Input: part model. Units: mm. Frame: model coordinates. A direction names the side the tool comes from. Coordinates: 2 decimals unless noted, no trailing zeros. Write each loop counter-clockwise with the first axis right and the second up, starting at its lowest first coordinate (ties: lowest second). Pieces come first, ordered by that corner, then holes.
1) Section query B-B (y = -1). Output: boundary loops of the cut face in (x, z).
2) Pin query (flat end, axial travel): pin 1 Ø6.5 at (y, z) = (67.5, -52.5) entering from -X. Return the tip coordinate at first contact, or that it passes through.
3) Line query: L1, parallel to Z at x = 1.55, y = -185; L2, parallel to Z at x = -22, y = 141.5; L3, parallel to Y at x = -14.5, z = 13.5. Output: solid intervals per line, ascending.
4) Draft query along X for faces 4 (the flat face through (0.5, 185, -65)), 5 (the flat face through (-13, -3, -60)), 6 (the flat face through (0, -175, -54)), 7 (the flat face through (0.5, -185, -65)). Return one class per face: pulls with the +X half, pulls with the -X half, needs draft (parallel to the pull), parting line crosses it, or undercut.
5) Set-up query: faces 1 (the cylindrical face through (1.565, 188.075, 64.317)), 2 (the flat face through (-13, 190, -1)), 3 (the flat face through (0, -60, -54)). Return all of +Z, -Z, +X, -X, +Y, -Y with unobstructed straight access to the full face (end or side cutting, diameter ignored); none if empty.
6) Section query A-A (x = -18.5). Output: boundary loops of the cut face in (y, z).
7) Section query C-C (z = 17). Output: boundary loops of the cut face in (x, y), then the cut area to 3 significant figures.
from build123d import *

# Parameters (mm, degrees)
SKETCH1_W                        = 380
SKETCH1_H                        = 140
SKETCH1_W_2                      = 360
SKETCH1_H_2                      = 120
SKETCH1_R                        = 2
BOSS_EXTRUDE2_DEPTH              = 3
SKETCH1_6_W                      = 380
SKETCH1_6_H                      = 140
SKETCH1_6_W_2                    = 360
SKETCH1_6_H_2                    = 120
BOSS_EXTRUDE5_DEPTH              = 29
SKETCH14_W                       = 378
SKETCH14_H                       = 138
SKETCH14_W_2                     = 377.2
SKETCH14_H_2                     = 137.2
BOSS_EXTRUDE7_DEPTH              = 0.2
SKETCH14_4_R                     = 3.95
BOSS_EXTRUDE9_DEPTH              = 0.8
MOUNTING_MAGNET_HOLES_DEPTH      = 0.6
MOUNTING_MAGNET_HOLES_DEPTH_BACK = 1.5
SKETCH14_5_R                     = 3.15
SKETCH17_W                       = 378.4
SKETCH17_H                       = 138.4
SKETCH17_W_2                     = 377.2
SKETCH17_H_2                     = 137.2
BOSS_EXTRUDE10_DEPTH             = 0.4
CHAMFER1_SIZE                    = 0.4
CHAMFER1_SIZE_2                  = 0.230940108
COVER_START                      = -0.4
SKETCH18_R                       = 3.15
COVER_MAGNET_HOLES_DEPTH         = 2.1


with BuildPart() as part:
    # Sketch1 → Boss-Extrude2 (new body)
    # profile 1 of 13: a face of its own
    with BuildSketch(Plane.YZ):
        Rectangle(SKETCH1_W, SKETCH1_H)
        Rectangle(SKETCH1_W_2, SKETCH1_H_2, mode=Mode.SUBTRACT)
    # profile 2 of 13: a face of its own
    with BuildSketch(Plane.YZ):
        with BuildLine():
            Line((-180, 60), (-180, 48))
            Line((-180, 48), (-174, 48))
            ThreePointArc((-174, 48), (-169.757359313, 49.757359313), (-168, 54))
            Line((-168, 54), (-168, 60))
            Line((-168, 60), (-180, 60))
        make_face()
        with Locations(Location((-172.5, 52.5, 0), (0, 0, 270))):
            Circle(SKETCH1_R, mode=Mode.SUBTRACT)
    # profile 3 of 13: a face of its own
    with BuildSketch(Plane.YZ):
        with BuildLine():
            Line((-60, 60), (-72, 60))
            Line((-72, 60), (-72, 54))
            ThreePointArc((-72, 54), (-70.242640687, 49.757359313), (-66, 48))
            Line((-66, 48), (-60, 48))
            Line((-60, 48), (-60, 60))
        make_face()
        with Locations(Location((-67.5, 52.5, 0), (0, 0, 270))):
            Circle(SKETCH1_R, mode=Mode.SUBTRACT)
    # profile 4 of 13: a face of its own
    with BuildSketch(Plane.YZ):
        with BuildLine():
            Line((-48, 60), (-60, 60))
            Line((-60, 60), (-60, 48))
            Line((-60, 48), (-54, 48))
            ThreePointArc((-54, 48), (-49.757359313, 49.757359313), (-48, 54))
            Line((-48, 54), (-48, 60))
        make_face()
        with Locations(Location((-52.5, 52.5, 0), (0, 0, 270))):
            Circle(SKETCH1_R, mode=Mode.SUBTRACT)
    # profile 5 of 13: a face of its own
    with BuildSketch(Plane.YZ):
        with BuildLine():
            Line((-60, -48), (-60, -60))
            Line((-60, -60), (-48, -60))
            Line((-48, -60), (-48, -54))
            ThreePointArc((-48, -54), (-49.757359313, -49.757359313), (-54, -48))
            Line((-54, -48), (-60, -48))
        make_face()
        with Locations(Location((-52.5, -52.5, 0), (0, 0, 270))):
            Circle(SKETCH1_R, mode=Mode.SUBTRACT)
    # profile 6 of 13: a face of its own
    with BuildSketch(Plane.YZ):
        with BuildLine():
            Line((-72, -54), (-72, -60))
            Line((-72, -60), (-60, -60))
            Line((-60, -60), (-60, -48))
            Line((-60, -48), (-66, -48))
            ThreePointArc((-66, -48), (-70.242640687, -49.757359313), (-72, -54))
        make_face()
        with Locations(Location((-67.5, -52.5, 0), (0, 0, 270))):
            Circle(SKETCH1_R, mode=Mode.SUBTRACT)
    # profile 7 of 13: a face of its own
    with BuildSketch(Plane.YZ):
        with BuildLine():
            Line((-180, -48), (-180, -60))
            Line((-180, -60), (-168, -60))
            Line((-168, -60), (-168, -54))
            ThreePointArc((-168, -54), (-169.757359313, -49.757359313), (-174, -48))
            Line((-174, -48), (-180, -48))
        make_face()
        with Locations(Location((-172.5, -52.5, 0), (0, 0, 270))):
            Circle(SKETCH1_R, mode=Mode.SUBTRACT)
    # profile 8 of 13: a face of its own
    with BuildSketch(Plane.YZ):
        with BuildLine():
            Line((48, -54), (48, -60))
            Line((48, -60), (60, -60))
            Line((60, -60), (60, -48))
            Line((60, -48), (54, -48))
            ThreePointArc((54, -48), (49.757359313, -49.757359313), (48, -54))
        make_face()
        with Locations(Location((52.5, -52.5, 0), (0, 0, 270))):
            Circle(SKETCH1_R, mode=Mode.SUBTRACT)
    # profile 9 of 13: a face of its own
    with BuildSketch(Plane.YZ):
        with BuildLine():
            Line((60, -48), (60, -60))
            Line((60, -60), (72, -60))
            Line((72, -60), (72, -54))
            ThreePointArc((72, -54), (70.242640687, -49.757359313), (66, -48))
            Line((66, -48), (60, -48))
        make_face()
        with Locations(Location((67.5, -52.5, 0), (0, 0, 270))):
            Circle(SKETCH1_R, mode=Mode.SUBTRACT)
    # profile 10 of 13: a face of its own
    with BuildSketch(Plane.YZ):
        with BuildLine():
            Line((72, 60), (60, 60))
            Line((60, 60), (60, 48))
            Line((60, 48), (66, 48))
            ThreePointArc((66, 48), (70.242640687, 49.757359313), (72, 54))
            Line((72, 54), (72, 60))
        make_face()
        with Locations(Location((67.5, 52.5, 0), (0, 0, 270))):
            Circle(SKETCH1_R, mode=Mode.SUBTRACT)
    # profile 11 of 13: a face of its own
    with BuildSketch(Plane.YZ):
        with BuildLine():
            Line((60, 60), (48, 60))
            Line((48, 60), (48, 54))
            ThreePointArc((48, 54), (49.757359313, 49.757359313), (54, 48))
            Line((54, 48), (60, 48))
            Line((60, 48), (60, 60))
        make_face()
        with Locations(Location((52.5, 52.5, 0), (0, 0, 270))):
            Circle(SKETCH1_R, mode=Mode.SUBTRACT)
    # profile 12 of 13: a face of its own
    with BuildSketch(Plane.YZ):
        with BuildLine():
            Line((174, 48), (180, 48))
            Line((180, 48), (180, 60))
            Line((180, 60), (168, 60))
            Line((168, 60), (168, 54))
            ThreePointArc((168, 54), (169.757359313, 49.757359313), (174, 48))
        make_face()
        with Locations(Location((172.5, 52.5, 0), (0, 0, 270))):
            Circle(SKETCH1_R, mode=Mode.SUBTRACT)
    # profile 13 of 13: a face of its own
    with BuildSketch(Plane.YZ):
        with BuildLine():
            Line((168, -54), (168, -60))
            Line((168, -60), (180, -60))
            Line((180, -60), (180, -48))
            Line((180, -48), (174, -48))
            ThreePointArc((174, -48), (169.757359313, -49.757359313), (168, -54))
        make_face()
        with Locations(Location((172.5, -52.5, 0), (0, 0, 270))):
            Circle(SKETCH1_R, mode=Mode.SUBTRACT)
    extrude(amount=BOSS_EXTRUDE2_DEPTH)

    # Sketch1<6> → Boss-Extrude5 (add)
    with BuildSketch(Plane.YZ):
        Rectangle(SKETCH1_6_W, SKETCH1_6_H)
        Rectangle(SKETCH1_6_W_2, SKETCH1_6_H_2, mode=Mode.SUBTRACT)
    extrude(amount=-BOSS_EXTRUDE5_DEPTH)

    # Sketch14 → Boss-Extrude7 (add)
    with BuildSketch(Plane(origin=(-29, 0, 0), x_dir=(0, -1, 0), z_dir=(-1, 0, 0))):
        Rectangle(SKETCH14_W, SKETCH14_H)
        Rectangle(SKETCH14_W_2, SKETCH14_H_2, mode=Mode.SUBTRACT)
    extrude(amount=BOSS_EXTRUDE7_DEPTH)

    # Sketch14<4> → Boss-Extrude9 (add)
    with BuildSketch(Plane(origin=(-29, 0, 0), x_dir=(0, -1, 0), z_dir=(-1, 0, 0))):
        with Locations(Location((-182.928932188, 62.928932188, 0), (0, 0, 270))):
            Circle(SKETCH14_4_R)
        with Locations(Location((182.928932188, 62.928932188, 0), (0, 0, 270))):
            Circle(SKETCH14_4_R)
        with Locations(Location((182.928932188, -62.928932188, 0), (0, 0, 270))):
            Circle(SKETCH14_4_R)
        with Locations(Location((-182.928932188, -62.928932188, 0), (0, 0, 270))):
            Circle(SKETCH14_4_R)
    extrude(amount=BOSS_EXTRUDE9_DEPTH)

    # Sketch14<5> → Mounting magnet holes (cut, two sides: drawn at the far end of the back side and taken through both)
    with BuildSketch(Plane(origin=(-29, 0, 0), x_dir=(0, -1, 0), z_dir=(-1, 0, 0)).offset(-MOUNTING_MAGNET_HOLES_DEPTH_BACK)):
        with Locations(Location((-182.928932188, 62.928932188, 0), (0, 0, 90))):
            Circle(SKETCH14_5_R)
        with Locations(Location((182.928932188, 62.928932188, 0), (0, 0, 270))):
            Circle(SKETCH14_5_R)
        with Locations(Location((182.928932188, -62.928932188, 0), (0, 0, 90))):
            Circle(SKETCH14_5_R)
        with Locations(Location((-182.928932188, -62.928932188, 0), (0, 0, 270))):
            Circle(SKETCH14_5_R)
    extrude(amount=MOUNTING_MAGNET_HOLES_DEPTH + MOUNTING_MAGNET_HOLES_DEPTH_BACK, mode=Mode.SUBTRACT)

    # Sketch17 → Boss-Extrude10 (add)
    with BuildSketch(Plane(origin=(-29.2, 0, 0), x_dir=(0, -1, 0), z_dir=(-1, 0, 0))):
        Rectangle(SKETCH17_W, SKETCH17_H)
        Rectangle(SKETCH17_W_2, SKETCH17_H_2, mode=Mode.SUBTRACT)
    extrude(amount=BOSS_EXTRUDE10_DEPTH)

    # Chamfer1
    # the kernel refuses this chamfer: 0.4, 0.230940108 mm, written as the material it takes off along each edge
    with BuildSketch(Plane(origin=(-29.6, 190.234834302, -69.2), x_dir=(0.9998132206222082, 0, -0.01932676561269006), z_dir=(0, -1, 0))) as chamfer1_piece_1:
        Polygon((CHAMFER1_SIZE * 0.999813220622, CHAMFER1_SIZE * 0.0193267656127), (-CHAMFER1_SIZE_2 * 0.0193267655856, CHAMFER1_SIZE_2 * 0.999813219219), (0, 0), align=None)
    extrude(amount=380.469668604, mode=Mode.SUBTRACT)
    with BuildSketch(Plane(origin=(-29.6, -189.2, -70.234834302), x_dir=(-0.057893862402669215, 0.9983227437537926, 0), z_dir=(0, 0, 1)), Plane(origin=(-29.6, 189.2, 70.234834302), x_dir=(-0.057893862402669215, -0.9983227437537926, 0), z_dir=(0, 0, -1))) as chamfer1_piece_2:
        Polygon((CHAMFER1_SIZE_2 * 0.998322742353, -CHAMFER1_SIZE_2 * 0.0578938623214), (-CHAMFER1_SIZE * 0.0578938624027, -CHAMFER1_SIZE * 0.998322743754), (0, 0), align=None)
    extrude(amount=140.469668604, mode=Mode.SUBTRACT)
    with BuildSketch(Plane(origin=(-29.6, -190.234834302, 69.2), x_dir=(-0.057893862402672656, 0, -0.9983227437537925), z_dir=(0, 1, 0))) as chamfer1_piece_3:
        Polygon((CHAMFER1_SIZE_2 * 0.998322742353, -CHAMFER1_SIZE_2 * 0.0578938623214), (-CHAMFER1_SIZE * 0.0578938624027, -CHAMFER1_SIZE * 0.998322743754), (0, 0), align=None)
    extrude(amount=380.469668604, mode=Mode.SUBTRACT)

    # Sketch18 → Cover magnet holes (cut)
    with BuildSketch(Plane.YZ.offset(3).offset(COVER_START)):
        with Locations(Location((-185, 65, 0), (0, 0, 270))):
            Circle(SKETCH18_R)
        with Locations(Location((185, 65, 0), (0, 0, 90))):
            Circle(SKETCH18_R)
        with Locations(Location((185, -65, 0), (0, 0, 270))):
            Circle(SKETCH18_R)
        with Locations(Location((-185, -65, 0), (0, 0, 90))):
            Circle(SKETCH18_R)
    extrude(amount=-COVER_MAGNET_HOLES_DEPTH, mode=Mode.SUBTRACT)


solid = part.part
Answer:
1. outline: (-29.6, -68.97) - (-29.2, -69.2) - (-29.2, -69) - (-29, -69) - (-29, -70) - (3, -70) - (3, -60) - (-29, -60) - (-29, -68.6) - (-29.6, -68.6) - close; (-29.6, 68.6) - (-29, 68.6) - (-29, 60) - (3, 60) - (3, 70) - (-29, 70) - (-29, 69) - (-29.2, 69) - (-29.2, 69.2) - (-29.6, 68.97) - close
2. pin 1: stops at x = 0
3. L1: z = -70 to -68.15, -61.85 to 61.85, 68.15 to 70
3. L2: z = -70 to -60, 60 to 70
3. L3: y = -190 to -180, 180 to 190
4. face 4: undercut
4. face 5: needs draft
4. face 6: pulls with the -X half
4. face 7: undercut
5. face 1: none
5. face 2: +Z, -Z, +X, -X, +Y
5. face 3: -X
6. outline: (-190, -70) - (190, -70) - (190, 70) - (-190, 70) - close; hole (-180, -60) - (180, -60) - (180, 60) - (-180, 60) - close
7. outline: (-29.6, -188.97) - (-29.2, -189.2) - (-29.2, -189) - (-29, -189) - (-29, -190) - (3, -190) - (3, -180) - (-29, -180) - (-29, -188.6) - (-29.6, -188.6) - close; (-29.6, 188.6) - (-29, 188.6) - (-29, 180) - (3, 180) - (3, 190) - (-29, 190) - (-29, 189) - (-29.2, 189) - (-29.2, 189.2) - (-29.6, 188.97) - close
7. area: 641 mm2
